For this review, use the dimensioned drawing (mm, ordinates from the lowest corner) and the shaded views. Coordinates: 2 decimals unless noted, no trailing zeros. Loops run counter-clockwise (first coordinate to the right, second up) from the corner with the lowest first, then second, coordinate; pieces in that order, holes last.
1. Take a section at B-B, the plane x = 56.5. State the section outline as (y, z) points.
2. Clearance check with flat-ended pins moving along their axes: P1, Ø10, axis at x = 63.5, z = 35, coming from the +Y side; P2, Ø1, axis at y = 23, z = 14.5, coming from the +X side; P3, Ø1, axis at x = 30.5, z = 39, coming from the -Y side. State where each tip first meets the part, or that it passes through.
3. Take a section at A-A, the plane z = 13. State the section outline as (x, y) points.
4. To check wall thickness, follow probe 1 along Y at (x, z) = (16.5, 5.5); probe 2 along Z at (x, y) = (16.5, 42); probe 3 along Z at (x, y) = (42.5, 48). State the ranges of each line that lie inside material, in increasing order.
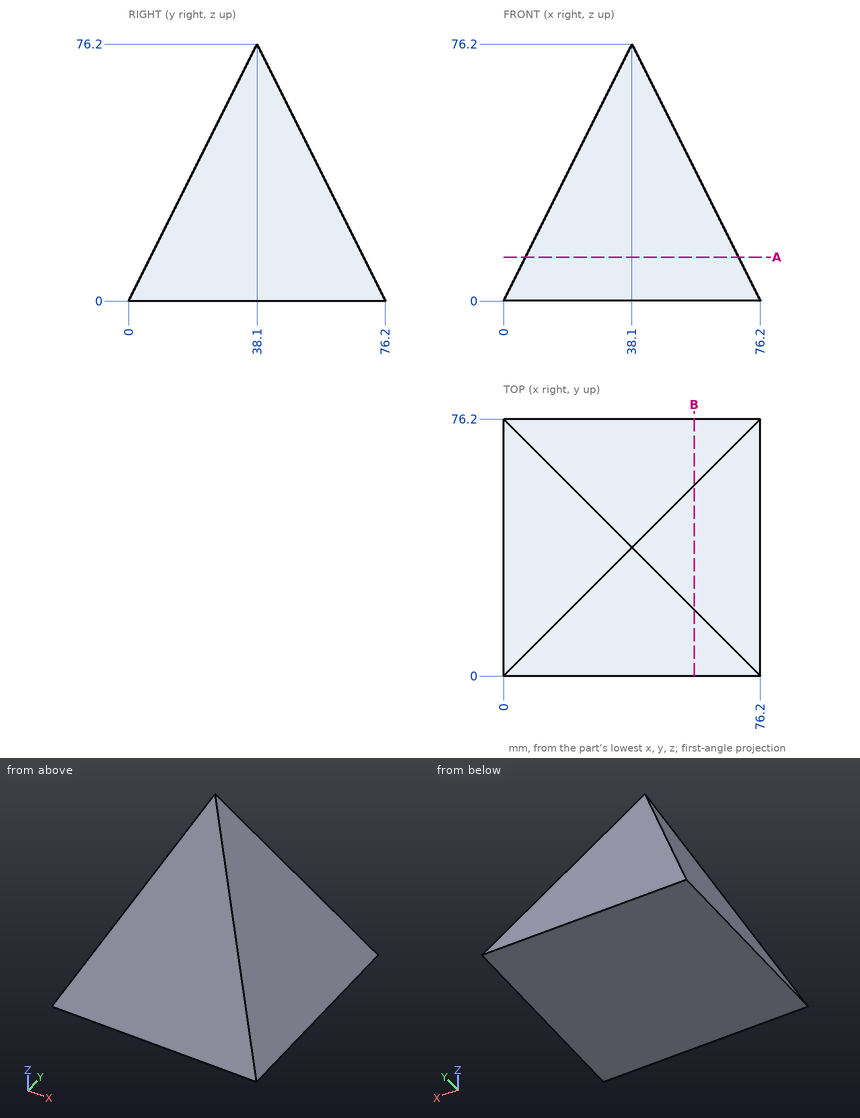
Results list:
1. outline: (0, 0) - (76.2, 0) - (56.5, 39.4) - (19.7, 39.4) - close
2. P1: stops at y = 60.81
2. P2: stops at x = 69.2
2. P3: stops at y = 19.25
3. outline: (6.5, 6.5) - (69.7, 6.5) - (69.7, 69.7) - (6.5, 69.7) - close
4. probe 1: y = 2.75 to 73.45
4. probe 2: z = 0 to 33
4. probe 3: z = 0 to 56.4
